```python
from build123d import *
from build123d.topology import SkipClean

# Parameters (mm, degrees)
BOSS_EXTRUDE3_DEPTH = 37
CUT_EXTRUDE3_REACH  = 132.806
SKETCH3_R           = 11.5
CUT_EXTRUDE4_REACH  = 132.806
SKETCH4_R           = 1.25
SKETCH6_W           = 38
SKETCH6_H           = 23
CUT_EXTRUDE6_DEPTH  = 3
SKETCH10_W          = 3
SKETCH10_H          = 23
BOSS_EXTRUDE5_DEPTH = 7.5
CUT_EXTRUDE11_REACH = 130.329
SKETCH11_R          = 1.25
SKETCH12_R          = 2.05
CUT_EXTRUDE12_DEPTH = 3
CUT_EXTRUDE13_REACH = 132.806
SKETCH13_R          = 4
FILLET5_SIZE        = 15
SKETCH14_R          = 1.25
BOSS_EXTRUDE6_DEPTH = 7
CUT_EXTRUDE14_REACH = 136.318
SKETCH15_R          = 1.25
SKETCH16_R          = 2.55
CUT_EXTRUDE15_DEPTH = 4


with BuildPart() as part:
    # Sketch2 → Boss-Extrude3 (new body)
    with BuildSketch(Plane(origin=(0, 0, 0), x_dir=(1, 0, 0), z_dir=(0, 1, 0))):
        Polygon((0, 0), (0, -63), (108.5, -63), (108.5, 0), (103.5, 0), (103.5, -58), (5, -58), (5, 0), align=None)
    extrude(amount=BOSS_EXTRUDE3_DEPTH)

    # Sketch3 → Cut-Extrude3 (cut, up to next)
    with BuildSketch(Plane.ZY, mode=Mode.PRIVATE) as cut_extrude3_sk1:
        with Locations((16, 18.5)):
            Circle(SKETCH3_R)
    cut_extrude3_tool1 = extrude(cut_extrude3_sk1.sketch, amount=-CUT_EXTRUDE3_REACH, mode=Mode.PRIVATE) & part.part
    add(cut_extrude3_tool1.solids().sort_by_distance((0, 18.5, 16))[0], mode=Mode.SUBTRACT)

    # Sketch4 → Cut-Extrude4 (cut, up to next)
    with BuildSketch(Plane.ZY, mode=Mode.PRIVATE) as cut_extrude4_sk1:
        with Locations((22.64, 32.19)):
            Circle(SKETCH4_R)
    cut_extrude4_tool1 = extrude(cut_extrude4_sk1.sketch, amount=-CUT_EXTRUDE4_REACH, mode=Mode.PRIVATE) & part.part
    # Sketch4 → Cut-Extrude4 (cut, up to next)
    with BuildSketch(Plane.ZY, mode=Mode.PRIVATE) as cut_extrude4_sk2:
        with Locations((30.64, 32.19)):
            Circle(SKETCH4_R)
    cut_extrude4_tool2 = extrude(cut_extrude4_sk2.sketch, amount=-CUT_EXTRUDE4_REACH, mode=Mode.PRIVATE) & part.part
    # Sketch4 → Cut-Extrude4 (cut, up to next)
    with BuildSketch(Plane.ZY, mode=Mode.PRIVATE) as cut_extrude4_sk3:
        with Locations((38.64, 32.19)):
            Circle(SKETCH4_R)
    cut_extrude4_tool3 = extrude(cut_extrude4_sk3.sketch, amount=-CUT_EXTRUDE4_REACH, mode=Mode.PRIVATE) & part.part
    # Sketch4 → Cut-Extrude4 (cut, up to next)
    with BuildSketch(Plane.ZY, mode=Mode.PRIVATE) as cut_extrude4_sk4:
        with Locations((46.64, 32.19)):
            Circle(SKETCH4_R)
    cut_extrude4_tool4 = extrude(cut_extrude4_sk4.sketch, amount=-CUT_EXTRUDE4_REACH, mode=Mode.PRIVATE) & part.part
    # Sketch4 → Cut-Extrude4 (cut, up to next)
    with BuildSketch(Plane.ZY, mode=Mode.PRIVATE) as cut_extrude4_sk5:
        with Locations((46.64, 4.81)):
            Circle(SKETCH4_R)
    cut_extrude4_tool5 = extrude(cut_extrude4_sk5.sketch, amount=-CUT_EXTRUDE4_REACH, mode=Mode.PRIVATE) & part.part
    # Sketch4 → Cut-Extrude4 (cut, up to next)
    with BuildSketch(Plane.ZY, mode=Mode.PRIVATE) as cut_extrude4_sk6:
        with Locations((38.64, 4.81)):
            Circle(SKETCH4_R)
    cut_extrude4_tool6 = extrude(cut_extrude4_sk6.sketch, amount=-CUT_EXTRUDE4_REACH, mode=Mode.PRIVATE) & part.part
    # Sketch4 → Cut-Extrude4 (cut, up to next)
    with BuildSketch(Plane.ZY, mode=Mode.PRIVATE) as cut_extrude4_sk7:
        with Locations((30.64, 4.81)):
            Circle(SKETCH4_R)
    cut_extrude4_tool7 = extrude(cut_extrude4_sk7.sketch, amount=-CUT_EXTRUDE4_REACH, mode=Mode.PRIVATE) & part.part
    # Sketch4 → Cut-Extrude4 (cut, up to next)
    with BuildSketch(Plane.ZY, mode=Mode.PRIVATE) as cut_extrude4_sk8:
        with Locations((22.64, 4.81)):
            Circle(SKETCH4_R)
    cut_extrude4_tool8 = extrude(cut_extrude4_sk8.sketch, amount=-CUT_EXTRUDE4_REACH, mode=Mode.PRIVATE) & part.part
    # Sketch4 → Cut-Extrude4 (cut, up to next)
    with BuildSketch(Plane.ZY, mode=Mode.PRIVATE) as cut_extrude4_sk9:
        with Locations((52.14, 26.69)):
            Circle(SKETCH4_R)
    cut_extrude4_tool9 = extrude(cut_extrude4_sk9.sketch, amount=-CUT_EXTRUDE4_REACH, mode=Mode.PRIVATE) & part.part
    # Sketch4 → Cut-Extrude4 (cut, up to next)
    with BuildSketch(Plane.ZY, mode=Mode.PRIVATE) as cut_extrude4_sk10:
        with Locations((52.14, 10.31)):
            Circle(SKETCH4_R)
    cut_extrude4_tool10 = extrude(cut_extrude4_sk10.sketch, amount=-CUT_EXTRUDE4_REACH, mode=Mode.PRIVATE) & part.part
    add(cut_extrude4_tool1.solids().sort_by_distance((0, 32.19, 22.64))[0], mode=Mode.SUBTRACT)
    add(cut_extrude4_tool2.solids().sort_by_distance((0, 32.19, 30.64))[0], mode=Mode.SUBTRACT)
    add(cut_extrude4_tool3.solids().sort_by_distance((0, 32.19, 38.64))[0], mode=Mode.SUBTRACT)
    add(cut_extrude4_tool4.solids().sort_by_distance((0, 32.19, 46.64))[0], mode=Mode.SUBTRACT)
    add(cut_extrude4_tool5.solids().sort_by_distance((0, 4.81, 46.64))[0], mode=Mode.SUBTRACT)
    add(cut_extrude4_tool6.solids().sort_by_distance((0, 4.81, 38.64))[0], mode=Mode.SUBTRACT)
    add(cut_extrude4_tool7.solids().sort_by_distance((0, 4.81, 30.64))[0], mode=Mode.SUBTRACT)
    add(cut_extrude4_tool8.solids().sort_by_distance((0, 4.81, 22.64))[0], mode=Mode.SUBTRACT)
    add(cut_extrude4_tool9.solids().sort_by_distance((0, 26.69, 52.14))[0], mode=Mode.SUBTRACT)
    add(cut_extrude4_tool10.solids().sort_by_distance((0, 10.31, 52.14))[0], mode=Mode.SUBTRACT)

    # Sketch6 → Cut-Extrude6 (cut)
    with BuildSketch(Plane.ZY):
        with Locations((38, 18.5)):
            Rectangle(SKETCH6_W, SKETCH6_H)
    extrude(amount=-CUT_EXTRUDE6_DEPTH, mode=Mode.SUBTRACT)

    # Sketch10 → Boss-Extrude5 (add)
    with BuildSketch(Plane(origin=(0, 0, 57), x_dir=(-1, 0, 0), z_dir=(0, 0, -1))):
        with Locations((-1.5, 18.5)):
            Rectangle(SKETCH10_W, SKETCH10_H)
    extrude(amount=BOSS_EXTRUDE5_DEPTH)

    # Sketch11 → Cut-Extrude11 (cut, up to next)
    with BuildSketch(Plane(origin=(3, 0, 0), x_dir=(0, 0, -1), z_dir=(1, 0, 0)), mode=Mode.PRIVATE) as cut_extrude11_sk1:
        with Locations(Location((-52.14, 26.69, 0), (0, 0, 180))):
            Circle(SKETCH11_R)
    cut_extrude11_tool1 = extrude(cut_extrude11_sk1.sketch, amount=-CUT_EXTRUDE11_REACH, mode=Mode.PRIVATE) & part.part
    # Sketch11 → Cut-Extrude11 (cut, up to next)
    with BuildSketch(Plane(origin=(3, 0, 0), x_dir=(0, 0, -1), z_dir=(1, 0, 0)), mode=Mode.PRIVATE) as cut_extrude11_sk2:
        with Locations(Location((-52.14, 10.31, 0), (0, 0, 180))):
            Circle(SKETCH11_R)
    cut_extrude11_tool2 = extrude(cut_extrude11_sk2.sketch, amount=-CUT_EXTRUDE11_REACH, mode=Mode.PRIVATE) & part.part
    add(cut_extrude11_tool1.solids().sort_by_distance((3, 26.69, 52.14))[0], mode=Mode.SUBTRACT)
    add(cut_extrude11_tool2.solids().sort_by_distance((3, 10.31, 52.14))[0], mode=Mode.SUBTRACT)

    # Sketch12 → Cut-Extrude12 (cut)
    with BuildSketch(Plane(origin=(5, 0, 0), x_dir=(0, 0, -1), z_dir=(1, 0, 0))):
        with Locations((-52.14, 26.69)):
            Circle(SKETCH12_R)
        with Locations((-46.64, 32.19)):
            Circle(SKETCH12_R)
        with Locations((-38.64, 32.19)):
            Circle(SKETCH12_R)
        with Locations((-30.64, 32.19)):
            Circle(SKETCH12_R)
        with Locations((-22.64, 32.19)):
            Circle(SKETCH12_R)
        with Locations((-30.64, 4.81)):
            Circle(SKETCH12_R)
        with Locations((-22.64, 4.81)):
            Circle(SKETCH12_R)
        with Locations((-38.64, 4.81)):
            Circle(SKETCH12_R)
        with Locations((-46.64, 4.81)):
            Circle(SKETCH12_R)
        with Locations((-52.14, 10.31)):
            Circle(SKETCH12_R)
    extrude(amount=-CUT_EXTRUDE12_DEPTH, mode=Mode.SUBTRACT)

    # Sketch13 → Cut-Extrude13 (cut, up to next)
    with BuildSketch(Plane(origin=(108.5, 0, 0), x_dir=(0, 0, -1), z_dir=(1, 0, 0)), mode=Mode.PRIVATE) as cut_extrude13_sk1:
        with Locations((-16, 18.5)):
            Circle(SKETCH13_R)
    cut_extrude13_tool1 = extrude(cut_extrude13_sk1.sketch, amount=-CUT_EXTRUDE13_REACH, mode=Mode.PRIVATE) & part.part
    add(cut_extrude13_tool1.solids().sort_by_distance((108.5, 18.5, 16))[0], mode=Mode.SUBTRACT)

    # Fillet5
    # a fillet whose section is not a circle: 15 mm, written as the material it adds along each edge
    with BuildSketch(Plane(origin=(103.5, 0, 58), x_dir=(0, 0, -1), z_dir=(0, 1, 0))) as fillet5_piece_1:
        with BuildLine():
            Bezier((FILLET5_SIZE, 0), (0, 0), (0, FILLET5_SIZE), weights=[1, 0.538461538, 1])
            Line((0, FILLET5_SIZE), (0, 0))
            Line((0, 0), (FILLET5_SIZE, 0))
        make_face()
    extrude(amount=37)
    with BuildSketch(Plane(origin=(5, 0, 58), x_dir=(0, 0, -1), z_dir=(0, 1, 0))) as fillet5_piece_2_section:
        with BuildLine():
            Bezier((FILLET5_SIZE, 0), (0, 0), (0, -FILLET5_SIZE), weights=[1, 0.538461538, 1])
            Line((0, -FILLET5_SIZE), (0, 0))
            Line((0, 0), (FILLET5_SIZE, 0))
        make_face()
    fillet5_piece_2 = extrude(amount=37, mode=Mode.PRIVATE)
    fillet5_piece_2 = fillet5_piece_2 - Plane(origin=(5, 32.19, 46.64), x_dir=(0, 0, -1), z_dir=(1, 0, 0)) * Cylinder(2.05, 135, mode=Mode.PRIVATE)
    fillet5_piece_2 = fillet5_piece_2 - Plane(origin=(5, 26.69, 52.14), x_dir=(0, 0, -1), z_dir=(1, 0, 0)) * Cylinder(2.05, 135, mode=Mode.PRIVATE)
    fillet5_piece_2 = fillet5_piece_2 - Plane(origin=(5, 10.31, 52.14), x_dir=(0, 0, -1), z_dir=(1, 0, 0)) * Cylinder(2.05, 135, mode=Mode.PRIVATE)
    fillet5_piece_2 = fillet5_piece_2 - Plane(origin=(5, 4.81, 46.64), x_dir=(0, 0, -1), z_dir=(1, 0, 0)) * Cylinder(2.05, 135, mode=Mode.PRIVATE)
    add(fillet5_piece_2)

    # Sketch14 → Boss-Extrude6 (add)
    # profile 1 of 2: a face of its own
    with BuildSketch(Plane.XY.offset(63)):
        with BuildLine():
            Line((54.25, 27.75), (54.25, 29.5))
            ThreePointArc((54.25, 29.5), (43.25, 18.5), (54.25, 7.5))
            Line((54.25, 7.5), (54.25, 9.25))
            ThreePointArc((54.25, 9.25), (53, 10.5), (54.25, 11.75))
            Line((54.25, 11.75), (54.25, 25.25))
            ThreePointArc((54.25, 25.25), (53, 26.5), (54.25, 27.75))
        make_face()
        with Locations((46.25, 18.5)):
            Circle(SKETCH14_R, mode=Mode.SUBTRACT)
    # profile 2 of 2: a face of its own
    with BuildSketch(Plane.XY.offset(63)):
        with BuildLine():
            ThreePointArc((65.25, 18.5), (62.028174593, 26.278174593), (54.25, 29.5))
            Line((54.25, 29.5), (54.25, 27.75))
            ThreePointArc((54.25, 27.75), (55.133883476, 27.383883476), (55.5, 26.5))
            ThreePointArc((55.5, 26.5), (55.133883476, 25.616116524), (54.25, 25.25))
            Line((54.25, 25.25), (54.25, 11.75))
            ThreePointArc((54.25, 11.75), (55.133883476, 11.383883476), (55.5, 10.5))
            ThreePointArc((55.5, 10.5), (55.133883476, 9.616116524), (54.25, 9.25))
            Line((54.25, 9.25), (54.25, 7.5))
            ThreePointArc((54.25, 7.5), (62.028174593, 10.721825407), (65.25, 18.5))
        make_face()
        with Locations((62.25, 18.5)):
            Circle(SKETCH14_R, mode=Mode.SUBTRACT)
    extrude(amount=BOSS_EXTRUDE6_DEPTH)

    # Sketch15 → Cut-Extrude14 (cut, up to next)
    with BuildSketch(Plane.XY.offset(70), mode=Mode.PRIVATE) as cut_extrude14_sk1:
        with Locations((54.25, 10.5)):
            Circle(SKETCH15_R)
    cut_extrude14_tool1 = extrude(cut_extrude14_sk1.sketch, amount=-CUT_EXTRUDE14_REACH, mode=Mode.PRIVATE) & part.part
    # Sketch15 → Cut-Extrude14 (cut, up to next)
    with BuildSketch(Plane.XY.offset(70), mode=Mode.PRIVATE) as cut_extrude14_sk2:
        with Locations((46.25, 18.5)):
            Circle(SKETCH15_R)
    cut_extrude14_tool2 = extrude(cut_extrude14_sk2.sketch, amount=-CUT_EXTRUDE14_REACH, mode=Mode.PRIVATE) & part.part
    # Sketch15 → Cut-Extrude14 (cut, up to next)
    with BuildSketch(Plane.XY.offset(70), mode=Mode.PRIVATE) as cut_extrude14_sk3:
        with Locations((54.25, 26.5)):
            Circle(SKETCH15_R)
    cut_extrude14_tool3 = extrude(cut_extrude14_sk3.sketch, amount=-CUT_EXTRUDE14_REACH, mode=Mode.PRIVATE) & part.part
    # Sketch15 → Cut-Extrude14 (cut, up to next)
    with BuildSketch(Plane.XY.offset(70), mode=Mode.PRIVATE) as cut_extrude14_sk4:
        with Locations((62.25, 18.5)):
            Circle(SKETCH15_R)
    cut_extrude14_tool4 = extrude(cut_extrude14_sk4.sketch, amount=-CUT_EXTRUDE14_REACH, mode=Mode.PRIVATE) & part.part
    add(cut_extrude14_tool1.solids().sort_by_distance((54.25, 10.5, 70))[0], mode=Mode.SUBTRACT)
    add(cut_extrude14_tool2.solids().sort_by_distance((46.25, 18.5, 70))[0], mode=Mode.SUBTRACT)
    add(cut_extrude14_tool3.solids().sort_by_distance((54.25, 26.5, 70))[0], mode=Mode.SUBTRACT)
    add(cut_extrude14_tool4.solids().sort_by_distance((62.25, 18.5, 70))[0], mode=Mode.SUBTRACT)

    # Sketch16 → Cut-Extrude15 (cut)
    with SkipClean():  # the faces are left unmerged after this step: merging them gives an invalid solid
        with BuildSketch(Plane(origin=(0, 0, 58), x_dir=(-1, 0, 0), z_dir=(0, 0, -1))):
            with Locations((-46.25, 18.5)):
                Circle(SKETCH16_R)
            with Locations((-54.25, 10.5)):
                Circle(SKETCH16_R)
            with Locations((-62.25, 18.5)):
                Circle(SKETCH16_R)
            with Locations((-54.25, 26.5)):
                Circle(SKETCH16_R)
        extrude(amount=-CUT_EXTRUDE15_DEPTH, mode=Mode.SUBTRACT)


solid = part.part
```
For this review, take the finished solid that the model builds, in its own axes (mm). A direction names the side the tool comes from. Round coordinates to 2 decimals unless told otherwise and drop trailing zeros. Order: outer loops, then holes, each group sorted by start corner. A loop starts at its lowest first (then second) coordinate and runs counter-clockwise, first axis right, second up. Notation, with made-up numbers: (1, 73.5) -> (27, 73.5) arc R16 ccw to (27, 94.5) -> close; hole circle Ø6 at (-39, 47.5). An arc over 180 degrees is marked (long way). Use a Markdown table: item, result.
Item 1: Machinability: for faces 3 (the flat face through (55, 9, 62)), 4 (the flat face through (1, 30, 34)), 5 (the flat face through (2, 31, 32)), which of the approach directions +Z, -Z, +X, -X, +Y, -Y give a long, thin tool a straight path to every point of the face, cutting with its end or side? Answer none if there is none.
Resolved:
| item | result |
|---|---|
| face 3 | -Z |
| face 4 | -X |
| face 5 | none |
Item 2: For pin 1 (2 mm diameter, centred on x = 25, y = 28, fed in from -Z); pin 2 (12 mm diameter, centred on x = 85, y = 25.5, fed in from -Z); pin 3 (4 mm diameter, centred on x = 89.5, y = 11, fed in from -Z), all flat-tipped, find the tip position at first contact; note any pin that passes through.
Resolved:
| item | result |
|---|---|
| pin 1 | stops at z = 58 |
| pin 2 | stops at z = 57.67 |
| pin 3 | stops at z = 57.54 |
Item 3: Draft analysis for pull direction Y (two halves, no side actions). For faces 1 (the flat face through (46, 0, 59)), 2 (the cylindrical face through (56.8, 10.6, 60)), state which applies: +Y half, -Y half, draft (parallel to the pull), parting line (faces both ways), or undercut.
Resolved:
| item | result |
|---|---|
| face 1 | -Y half |
| face 2 | undercut |
Item 4: Take a section at B-B (x = 46.25). State the section outline as (y, z) points, plus the area to 3 significant figures.
Resolved:
| item | result |
|---|---|
| outline | (0, 58) -> (15.95, 58) -> (15.95, 62) -> (17.25, 62) -> (17.25, 70) -> (10.95, 70) -> (10.95, 63) -> (0, 63) -> close; (19.75, 62) -> (21.05, 62) -> (21.05, 58) -> (37, 58) -> (37, 63) -> (26.05, 63) -> (26.05, 70) -> (19.75, 70) -> close |
| area | 250 mm² |
Item 5: Take a section at C-C (z = 8). State the section outline as (x, y) points, plus the area to 3 significant figures.
Resolved:
| item | result |
|---|---|
| outline | (0, 0) -> (5, 0) -> (5, 10.24) -> (0, 10.24) -> close; (0, 26.76) -> (5, 26.76) -> (5, 37) -> (0, 37) -> close; (103.5, 0) -> (108.5, 0) -> (108.5, 37) -> (103.5, 37) -> close |
| area | 287 mm² |
Item 6: For line 1 along Y through (x, z) = (0.95, 52.14); line 2 along Y through (x, z) = (54.25, 62.8); line 3 along X through (y, z) = (23.5, 31.5), list the stretches that pass through material, from the lowest coordinate up. Write a range as [from, to].
Resolved:
| item | result |
|---|---|
| line 1 | y = [0, 9.06], [11.56, 25.44], [27.94, 37] |
| line 2 | y = [0, 9.25], [11.75, 25.25], [27.75, 37] |
| line 3 | x = [3, 5], [103.5, 108.5] |
Item 7: Take a section at A-A (z = 16). State the section outline as (x, y) points, plus the area to 3 significant figures.
Resolved:
| item | result |
|---|---|
| outline | (0, 0) -> (5, 0) -> (5, 7) -> (0, 7) -> close; (0, 30) -> (5, 30) -> (5, 37) -> (0, 37) -> close; (103.5, 0) -> (108.5, 0) -> (108.5, 14.5) -> (103.5, 14.5) -> close; (103.5, 22.5) -> (108.5, 22.5) -> (108.5, 37) -> (103.5, 37) -> close |
| area | 215 mm² |
Item 8: Take a section at D-D (y = 32.19). State how many separate pieces and enclosed holes the cut face has, plus the area to 3 significant figures.
Resolved:
| item | result |
|---|---|
| separate pieces | 5 |
| enclosed holes | 0 |
| area | 1,160 mm² |
